Can you work these out from the model? Positions are in its coordinate system, mm. Give positions to 0.01 mm unless a question says otherwise; leave off trailing zeros. Order: outer loops, then holes, each group sorted by start corner. A loop starts at its lowest first (then second) coordinate and runs counter-clockwise, first axis right, second up. Notation, with made-up numbers: (10.5, -14) - (39.5, -14) arc R17 cw to (39.5, -4) - close; hole circle Ø3 at (12.25, 55). An arc over 180 degrees is marked (long way). Return JSON: item names as keys, results as strings.
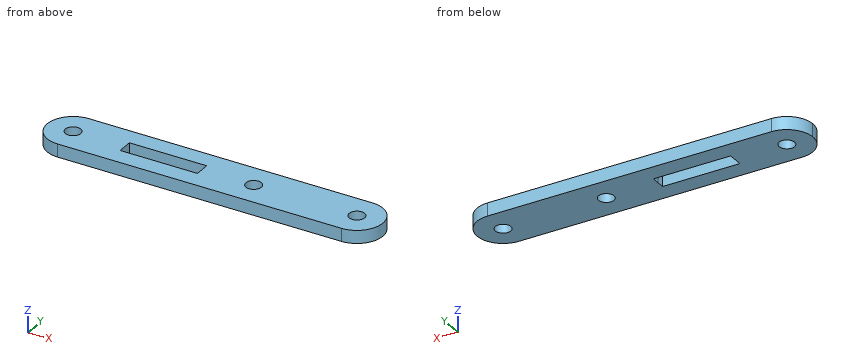
```python
from build123d import *

# Parameters (mm, degrees)
F0_R     = 1.5
F1_DEPTH = 2.5


with BuildPart() as f1:
    # F0 (on Top) → F1 (new body)
    with BuildSketch(Plane.XY):
        with BuildLine():
            Line((-16.842703, -5), (38.157297, -5))
            ThreePointArc((38.157297, -5), (43.157297, 0), (38.157297, 5))
            Line((38.157297, 5), (-16.842703, 5))
            ThreePointArc((-16.842703, 5), (-20.378237, 3.535534), (-21.842703, 0))
            ThreePointArc((-21.842703, 0), (-20.378237, -3.535534), (-16.842703, -5))
        make_face()
        with Locations((-16.842703, 0)):
            Circle(F0_R, mode=Mode.SUBTRACT)
        Polygon((-6.842703, -1.499771), (-6.842703, 0), (-6.842703, 1.499771), (8.131084, 1.499771), (8.157297, 0), (8.131084, -1.499771), align=None, mode=Mode.SUBTRACT)
        with Locations((18.157297, 0)):
            Circle(F0_R, mode=Mode.SUBTRACT)
        with BuildLine():
            ThreePointArc((36.657297, 0), (38.157297, 1.5), (39.657297, 0))
            ThreePointArc((39.657297, 0), (38.157297, -1.5), (36.657297, 0))
        make_face(mode=Mode.SUBTRACT)
    extrude(amount=F1_DEPTH)


solid = f1.part
```
1. Suppose I cut it at D-D (y = 4.25). List the corners of the cut face in (x, z) for me.
Checks:
{"outline": "(-19.48, 0) - (40.79, 0) - (40.79, 2.5) - (-19.48, 2.5) - close"}
2. Suppose I cut it at C-C (y = -2.5). List the corners of the cut face in (x, z) for me, plus the area to 3 significant figures.
Checks:
{"outline": "(-21.17, 0) - (42.49, 0) - (42.49, 2.5) - (-21.17, 2.5) - close", "area": "159 mm^2"}
3. For pin 1 Ø2.5 at (x, y) = (38.16, 0) entering from +Z; pin 2 Ø5 at (x, y) = (18.16, 0) entering from +Z; pin 3 Ø1 at (y, z) = (2.5, 2) entering from +X, each with a flat end and sliding along its axis, tell me the tip position at first contact or that it passes through.
Checks:
{"pin 1": "through", "pin 2": "z = 2.5", "pin 3": "x = 42.74"}
4. Suppose I cut it at A-A (x = -3). List the corners of the cut face in (y, z) for me.
Checks:
{"outline": "(-5, 0) - (-1.5, 0) - (-1.5, 2.5) - (-5, 2.5) - close; (1.5, 0) - (5, 0) - (5, 2.5) - (1.5, 2.5) - close"}
5. Suppose I cut it at B-B (z = 1.1). List the corners of the cut face in (x, y) for me.
Checks:
{"outline": "(-16.84, -5) - (38.16, -5) arc R5 ccw to (38.16, 5) - (-16.84, 5) arc R5 ccw to start; hole circle Ø3 at (-16.84, 0); hole (-6.84, -1.5) - (8.13, -1.5) - (8.16, 0) - (8.13, 1.5) - (-6.84, 1.5) - close; hole circle Ø3 at (18.16, 0); hole circle Ø3 at (38.16, 0)"}
6. If I drill on L1, parallel to X at y = 1, z = 0.25; L2, parallel to Y at x = -6, z = 1.9; L3, parallel to X at y = 0.25, z = 1.4, over which ranges is the centre line in solid material (lowest first)? Write a range as [from, to].
Checks:
{"L1": "[-21.74, -17.96], [-15.72, -6.84], [8.14, 17.04], [19.28, 37.04], [39.28, 43.06]", "L2": "[-5, -1.5], [1.5, 5]", "L3": "[-21.84, -18.32], [-15.36, -6.84], [8.15, 16.68], [19.64, 36.68], [39.64, 43.15]"}
